Part model, mm, in its own coordinate system. Face numbers are marked on the shaded views. A direction names the side the tool comes from. Coordinates: 2 decimals unless noted, no trailing zeros. Loops run counter-clockwise (first coordinate to the right, second up) from the corner with the lowest first, then second, coordinate; pieces in that order, holes last. Notation, with made-up numbers: (22.5, 76) - (79.5, 76) arc R29 cw to (79.5, 98) - close; hole circle Ø2 at (35.5, 80.25). An arc over 180 degrees is marked (long way). Use a Markdown table: item, result. Add a question column.
1. Wall check: probe 1 along Y at (x, z) = (-3, 5.25); probe 2 along Z at (x, y) = (13.25, -15.5); probe 3 along X at (y, z) = (-17.5, 8). Give the ranges that are in metal, low to high. Write a range as [from, to].
2. Drop flat-ended pins along their axis: pin 1 (3.5 mm diameter, centred on y = 0, z = -21, fed in from +X); pin 2 (4 mm diameter, centred on y = 15.5, z = -36.5, fed in from -X); pin 3 (4 mm diameter, centred on x = -1.5, y = 3, fed in from -Z). Give the stop position or say it passes through.
3. Band-saw the part on C-C, the plane x = -3. Give the cut face in (y, z), plus the area to 3 significant figures.
4. Band-saw the part on D-D, the plane y = 3. Give the cut face in (x, z).
5. Band-saw the part on A-A, the plane x = 0. Give the cut face in (y, z).
6. 3-axis set-ups, long thin cutter, end or side, ignore diameter. For the marked faces 1 and 2: which of +Z, -Z, +X, -X, +Y, -Y reach the whole face in a straight line?
7. Band-saw the part on B-B, the plane z = -21. Give the cut face in (x, y), plus the area to 3 significant figures.
from build123d import *

# Parameters (mm, degrees)
SKETCH_1_W          = 15
SKETCH_1_H          = 42
SKETCH_1_R          = 1.5
SKETCH_1_W_2        = 10
EXTRUDE_1_DEPTH     = 10
SKETCH_2_W          = 10
SKETCH_2_H          = 42
EXTRUDE_2_DEPTH     = 42
SKETCH_3_R          = 1.5
CUT_EXTRUDE_1_DEPTH = 15
FILLET_1_R          = 2
FILLET_2_R          = 5


with BuildPart() as part:
    # 草图1 → 凸台-拉伸1 (new body)
    # profile 1 of 2: a face of its own
    with BuildSketch(Plane.XY):
        Rectangle(SKETCH_1_W, SKETCH_1_H)
        Circle(SKETCH_1_R, mode=Mode.SUBTRACT)
        with Locations((3, -15)):
            Circle(SKETCH_1_R, mode=Mode.SUBTRACT)
        with Locations((3, 15)):
            Circle(SKETCH_1_R, mode=Mode.SUBTRACT)
        with Locations((-3, -15)):
            Circle(SKETCH_1_R, mode=Mode.SUBTRACT)
        with Locations((-3, 15)):
            Circle(SKETCH_1_R, mode=Mode.SUBTRACT)
    # profile 2 of 2: a face of its own
    with BuildSketch(Plane.XY):
        with Locations((12.5, 0)):
            Rectangle(SKETCH_1_W_2, SKETCH_1_H)
    extrude(amount=EXTRUDE_1_DEPTH)

    # 草图2 → 凸台-拉伸2 (add)
    with BuildSketch(Plane(origin=(0, 0, 0), x_dir=(-1, 0, 0), z_dir=(0, 0, -1))):
        with Locations((-12.5, 0)):
            Rectangle(SKETCH_2_W, SKETCH_2_H)
    extrude(amount=EXTRUDE_2_DEPTH)

    # 草图3 → 切除-拉伸1 (cut)
    with BuildSketch(Plane.ZY.offset(-7.5)):
        with Locations(Location((-36.5, 15.5, 0), (0, 0, 270))):
            Circle(SKETCH_3_R)
        with Locations(Location((-5.5, 15.5, 0), (0, 0, 270))):
            Circle(SKETCH_3_R)
        with Locations(Location((-36.5, -15.5, 0), (0, 0, 270))):
            Circle(SKETCH_3_R)
        with Locations(Location((-5.5, -15.5, 0), (0, 0, 270))):
            Circle(SKETCH_3_R)
        with Locations(Location((-21, 0, 0), (0, 0, 270))):
            Circle(SKETCH_3_R)
    extrude(amount=-CUT_EXTRUDE_1_DEPTH, mode=Mode.SUBTRACT)

    # 圆角1
    fillet_1_edges = [part.edges().sort_by_distance(p)[0] for p in [
        (7.5, 0, 0),
    ]]
    fillet(fillet_1_edges, radius=FILLET_1_R)

    # 圆角2
    fillet_2_edges = [part.edges().sort_by_distance(p)[0] for p in [
        (17.5, 0, 10),
    ]]
    fillet(fillet_2_edges, radius=FILLET_2_R)


solid = part.part
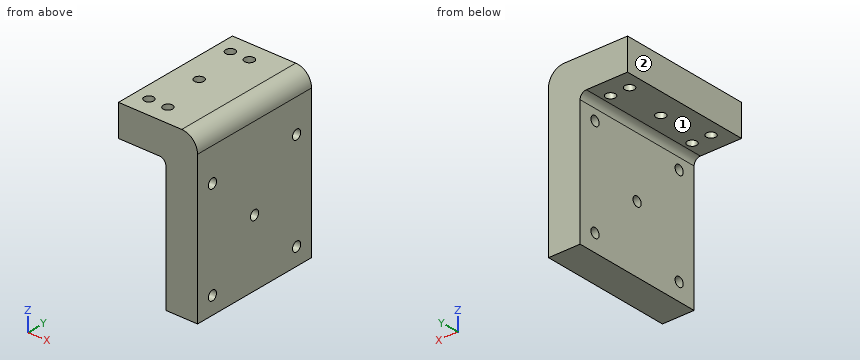
Geometry check:
| question | item | result |
|---|---|---|
| 1 | probe 1 | y = [-21, -16.5], [-13.5, 13.5], [16.5, 21] |
| 1 | probe 2 | z = [-42, -38], [-35, -7], [-4, 9.94] |
| 1 | probe 3 | x = [-7.5, 16.5] |
| 2 | pin 1 | stops at x = 17.5 |
| 2 | pin 2 | stops at x = 7.5 |
| 2 | pin 3 | stops at z = 0 |
| 3 | outline | (-21, 0) - (-16.5, 0) - (-16.5, 10) - (-21, 10) - close; (-13.5, 0) - (13.5, 0) - (13.5, 10) - (-13.5, 10) - close; (16.5, 0) - (21, 0) - (21, 10) - (16.5, 10) - close |
| 3 | area | 360 mm^2 |
| 4 | outline | (-7.5, 0) - (5.5, 0) arc R2 cw to (7.5, -2) - (7.5, -42) - (17.5, -42) - (17.5, 5) arc R5 ccw to (12.5, 10) - (-7.5, 10) - close |
| 5 | outline | (-21, 0) - (-1.5, 0) - (-1.5, 10) - (-21, 10) - close; (1.5, 0) - (21, 0) - (21, 10) - (1.5, 10) - close |
| 6 | face 1 | -Z, -X, +Y, -Y |
| 6 | face 2 | +Z, -Z, -X, +Y, -Y |
| 7 | outline | (7.5, -21) - (17.5, -21) - (17.5, -1.5) - (7.5, -1.5) - close; (7.5, 1.5) - (17.5, 1.5) - (17.5, 21) - (7.5, 21) - close |
| 7 | area | 390 mm^2 |
